The model under review builds one solid part; all positions refer to its coordinate system, in mm. A direction names the side the tool comes from. Round coordinates to 2 decimals unless told otherwise and drop trailing zeros. Order: outer loops, then holes, each group sorted by start corner. A loop starts at its lowest first (then second) coordinate and runs counter-clockwise, first axis right, second up.
```python
from build123d import *

# Parameters (mm, degrees)
F0_W      = 11.8
F0_H      = 22.5
F1_DEPTH  = 15.9
F2_W      = 11.8
F2_H      = 31.9
F3_DEPTH  = 2.5
F5_DEPTH  = 2.5
F6_DEPTH  = 22.7
F8_DEPTH  = 4
F9_R      = 2.33
F10_DEPTH = 3.2


with BuildPart() as f1:
    # F0 (on Top) → F1 (new body)
    with BuildSketch(Plane.XY):
        Rectangle(F0_W, F0_H)
    extrude(amount=F1_DEPTH)

    # F2 (on face) → F3 (join)
    with BuildSketch(Plane.XY.offset(15.9)):
        Rectangle(F2_W, F2_H)
    extrude(amount=F3_DEPTH)

    # F4 (on face) → F5 (cut)
    with BuildSketch(Plane.XY.offset(18.4)):
        with BuildLine():
            ThreePointArc((-0.665, 14.3968433571), (-0.4092676386, 12.7375856205), (1, 13.65))
            ThreePointArc((1, 13.65), (0.9124143795, 14.0592676386), (0.665, 14.3968433571))
            Line((0.665, 14.3968433571), (0.665, 13.65))
            Line((0.665, 13.65), (-0.665, 13.65))
            Line((-0.665, 13.65), (-0.665, 14.3968433571))
        make_face()
        with BuildLine():
            Line((0.665, 13.65), (0.665, 14.3968433571))
            ThreePointArc((0.665, 14.3968433571), (0, 14.65), (-0.665, 14.3968433571))
            Line((-0.665, 14.3968433571), (-0.665, 13.65))
            Line((-0.665, 13.65), (0.665, 13.65))
        make_face()
        with BuildLine():
            ThreePointArc((-0.665, 14.3968433571), (0, 14.65), (0.665, 14.3968433571))
            Line((0.665, 14.3968433571), (0.665, 15.95))
            Line((0.665, 15.95), (-0.665, 15.95))
            Line((-0.665, 15.95), (-0.665, 14.3968433571))
        make_face()
        with BuildLine():
            ThreePointArc((0.665, -14.3968433571), (0.9124143795, -14.0592676386), (1, -13.65))
            ThreePointArc((1, -13.65), (-0.4092676386, -12.7375856205), (-0.665, -14.3968433571))
            Line((-0.665, -14.3968433571), (-0.665, -13.65))
            Line((-0.665, -13.65), (0.665, -13.65))
            Line((0.665, -13.65), (0.665, -14.3968433571))
        make_face()
        with BuildLine():
            Line((-0.665, -13.65), (-0.665, -14.3968433571))
            ThreePointArc((-0.665, -14.3968433571), (0, -14.65), (0.665, -14.3968433571))
            Line((0.665, -14.3968433571), (0.665, -13.65))
            Line((0.665, -13.65), (-0.665, -13.65))
        make_face()
        with BuildLine():
            ThreePointArc((0.665, -14.3968433571), (0, -14.65), (-0.665, -14.3968433571))
            Line((-0.665, -14.3968433571), (-0.665, -15.95))
            Line((-0.665, -15.95), (0.665, -15.95))
            Line((0.665, -15.95), (0.665, -14.3968433571))
        make_face()
    extrude(amount=-F5_DEPTH, mode=Mode.SUBTRACT)

    # F0 (on Top) → F6 (join)
    with BuildSketch(Plane.XY):
        Rectangle(F0_W, F0_H)
    extrude(amount=F6_DEPTH)

    # F7 (on face) → F8 (join)
    with BuildSketch(Plane.XY.offset(22.7)):
        with BuildLine():
            ThreePointArc((-5.9, 5.35), (0, -0.55), (5.9, 5.35))
            ThreePointArc((5.9, 5.35), (4.171930009, 9.521930009), (0, 11.25))
            ThreePointArc((0, 11.25), (-4.171930009, 9.521930009), (-5.9, 5.35))
        make_face()
    extrude(amount=F8_DEPTH)

    # F9 (on face) → F10 (join)
    with BuildSketch(Plane.XY.offset(26.7)):
        with Locations((0, 5.35)):
            Circle(F9_R)
    extrude(amount=F10_DEPTH)


solid = f1.part
```
(1) To check wall thickness, follow probe 1 along X at (y, z) = (13.65, 16.5); probe 2 along Y at (x, z) = (-0.25, 21.75); probe 3 along Y at (x, z) = (0, 16.9). State the ranges of each line that lie inside material, in increasing order.
Data:
probe 1: x = -5.9 to -1, 1 to 5.9
probe 2: y = -11.25 to 11.25
probe 3: y = -12.65 to 12.65
(2) Consider section A-A (x = 3.75). Write out the cut boundary in (y, z).
Data:
outline: (-15.95, 15.9) - (-11.25, 15.9) - (-11.25, 0) - (11.25, 0) - (11.25, 15.9) - (15.95, 15.9) - (15.95, 18.4) - (11.25, 18.4) - (11.25, 22.7) - (9.9, 22.7) - (9.9, 26.7) - (0.8, 26.7) - (0.8, 22.7) - (-11.25, 22.7) - (-11.25, 18.4) - (-15.95, 18.4) - close
(3) Consider section D-D (x = -5). Write out the cut boundary in (y, z).
Data:
outline: (-15.95, 15.9) - (-11.25, 15.9) - (-11.25, 0) - (11.25, 0) - (11.25, 15.9) - (15.95, 15.9) - (15.95, 18.4) - (11.25, 18.4) - (11.25, 22.7) - (8.48, 22.7) - (8.48, 26.7) - (2.22, 26.7) - (2.22, 22.7) - (-11.25, 22.7) - (-11.25, 18.4) - (-15.95, 18.4) - close
(4) Insertion check: pin 1 (2.5 mm diameter, centred on x = -2.5, y = -13, fed in from +Z); pin 2 (3.5 mm diameter, centred on x = 1, y = -6, fed in from +Z); pin 3 (4 mm diameter, centred on x = -3.5, z = 20.5, fed in from +Y); pin 4 (1.8 mm diameter, centred on x = 0, y = -13.65, fed in from -Z). Each pin has a flat end and moves straight along its axis. Give the tip position at first contact, or say it passes through.
Data:
pin 1: stops at z = 18.4
pin 2: stops at z = 22.7
pin 3: stops at y = 11.25
pin 4: passes through
(5) Consider section B-B (y = 8.5). Write out the cut boundary in (x, z), and give its area (3 significant figures).
Data:
outline: (-5.9, 0) - (5.9, 0) - (5.9, 22.7) - (4.99, 22.7) - (4.99, 26.7) - (-4.99, 26.7) - (-4.99, 22.7) - (-5.9, 22.7) - close
area: 308 mm2
(6) For faces 1 (the flat face through (-1.4, 13.6, 18.4)), 2 (the flat face through (0, 11.25, 8)), 3 (the flat face through (-0.1, -12.5, 18.4)), 4 (the cylindrical face through (-0.259, -0.544, 24.672)), 5 (the flat face through (0, -11.25, 8)), list the 3-axis set-ups (+Z, -Z, +X, -X, +Y, -Y) from which the entire face can be reached by the end or side of a thin tool; tool diameter is ignored.
Data:
face 1: +Z, +X, -X, +Y
face 2: -Z, +X, -X, +Y
face 3: +Z, +X, -X, -Y
face 4: +Z
face 5: -Z, +X, -X, -Y
(7) Consider section C-C (z = 14). Write out the cut boundary in (x, y).
Data:
outline: (-5.9, -11.25) - (5.9, -11.25) - (5.9, 11.25) - (-5.9, 11.25) - close
